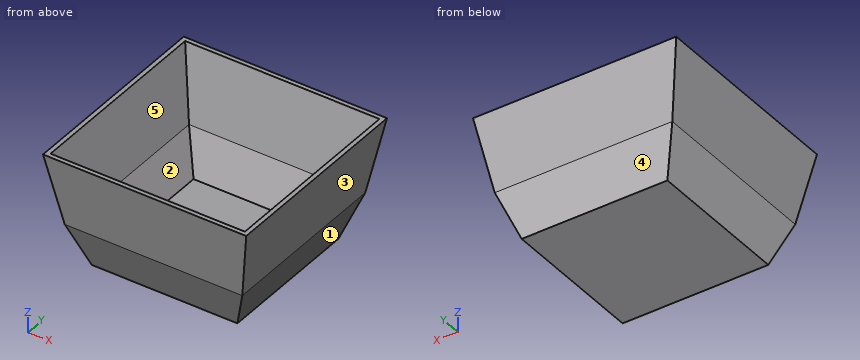
Autodesk Fusion 360 part; units mm, degrees
sketch "스케치1" plane through (0, 0, 0) normal (0, 0, 1) x (1, 0, 0) in component "Component'"
  line L0 (-50, 50) -> (50, 50)
  line L1 (50, 50) -> (50, -50)
  line L2 (50, -50) -> (-50, -50)
  line L3 (-50, -50) -> (-50, 50)
  line L4 (-150, -30) -> (-65.8539, -30)
  line L5 (-65.8539, -30) -> (-94.1954, 36.1303)
  line L6 (-94.1954, 36.1303) -> (-70, 20)
  line L7 (-70, 20) -> (-80, 50)
extrude "돌출1" add sketch "스케치1" along normal blind 30 draft 20 in component "Component'"
extrude "돌출2" add 1 faces at (-20.3064, 20.3064, 30) along direction (0, 0, 1) blind 50 draft 10 in component "Component'"
shell "쉘1" thickness 3 removed faces 1 at (-23.2452, 23.2452, 80) in component "Component'"
component "Component'" placed x (1, 0, 0) y (0, 1, 0) z (0, 0, 1) at (0, 0, 0)
Check sheet for the modelled part. Datum: model origin and axes. Units: mm. Face numbers are marked on the shaded views. A direction names the side the tool comes from. Coordinates: 2 decimals unless noted, no trailing zeros. Write each loop counter-clockwise with the first axis right and the second up, starting at its lowest first coordinate (ties: lowest second). Pieces come first, ordered by that corner, then holes. Notation, with made-up numbers: M -31.5,-2.75 L -5.5,-2.75 A21 ccw -5.5,20.25 Z; hole C 18,86 d11. An arc over 180 degrees is marked long. Write item = value, one per line. Start each with the question number.
1. Mould release check, pull along Y, two halves, no side actions. Record for the marked faces 3, 4 and 5: pulls with the +Y half, pulls with the -Y half, needs draft (parallel to the pull), parting line crosses it, or undercut.
2. Sectioned sample at D-D (z = 8.5). Record the cut outline in (x, y), then the cut area to 3 significant figures.
3. Go/stop test with flat-tipped pins: pin 1 (1.5 mm diameter, centred on x = -44.5, z = 16, fed in from +Y); pin 2 (6 mm diameter, centred on x = 30, y = 36.5, fed in from -Z); pin 3 (1.5 mm diameter, centred on y = -26, z = 51, fed in from +X); pin 4 (1 mm diameter, centred on y = 9.5, z = 65.5, fed in from +X). Record where each tip stops, or that it passes through.
4. Sectioned sample at B-B (z = 58). Record the cut outline in (x, y).
5. Tool access check on the marked faces 1 and 2. Record the directions out of +Z, -Z, +X, -X, +Y, -Y that give a thin tool (end or side, any length) a straight path to the whole face; none if there is none.
6. Sectioned sample at A-A (y = -13). Record the cut outline in (x, z).
7. Thickness scan on probe 1 along Z at (x, y) = (23.5, -3); probe 2 along X at (y, z) = (47, 18.5); probe 3 along Y at (x, z) = (-61, 77). Record the ranges inside material, lowest first.
The answers:
q1.face_3 = needs draft
q1.face_4 = pulls with the +Y half
q1.face_5 = undercut
q2.outline = M -53.09,-53.09 L 53.09,-53.09 L 53.09,53.09 L -53.09,53.09 Z; hole M -49.9,-49.9 L 49.9,-49.9 L 49.9,49.9 L -49.9,49.9 Z
q2.area = 1,320 mm²
q3.pin_1 = 56.1
q3.pin_2 = 0
q3.pin_3 = 64.75
q3.pin_4 = 67.27
q4.outline = M -65.86,-65.86 L 65.86,-65.86 L 65.86,65.86 L -65.86,65.86 Z; hole M -62.81,-62.81 L 62.81,-62.81 L 62.81,62.81 L -62.81,62.81 Z
q5.face_1 = -Z, +X, +Y, -Y
q5.face_2 = +Z
q6.outline = M -69.74,80 L -60.92,30 L -50,0 L 50,0 L 60.92,30 L 69.74,80 L 66.69,80 L 58.01,30.78 L 47.9,3 L -47.9,3 L -58.01,30.78 L -66.69,80 Z
q7.probe_1 = 0 to 3
q7.probe_2 = -56.73 to -53.54, 53.54 to 56.73
q7.probe_3 = -69.21 to -66.16, 66.16 to 69.21
